Autodesk Inventor part; units mm, degrees
ref_plane "YZ Plane" through (0, 0, 0) normal (1, 0, 0) x (0, 1, 0)
ref_plane "XZ Plane" through (0, 0, 0) normal (0, 1, 0) x (-1, 0, 0)
ref_plane "XY Plane" through (0, 0, 0) normal (0, 0, 1) x (1, 0, 0)
sketch "스케치1" plane through (0, 0, 0) normal (0, 1, 0) x (-1, 0, 0)
  line L0 (0, 0) -> (-315, 0)
  line L1 (-315, 0) -> (-315, -950)
  line L2 (-315, -950) -> (0, -950)
  line L3 (0, -950) -> (0, 0)
  line L4 (-315, -645) -> (-315, -475)
  line L5 (-315, -475) -> (-535, -475)
  line L6 (-535, -475) -> (-535, -645)
  line L7 (-535, -645) -> (-315, -645)
  line L8 (-315, -645) -> (-315, -475)
  line L9 (-315, -475) -> (-535, -475)
  line L10 (-315, -305) -> (-315, -475)
  line L11 (-315, -475) -> (-535, -475)
  line L12 (-535, -475) -> (-535, -305)
  line L13 (-535, -305) -> (-315, -305)
  line L14 (-315, -305) -> (-315, -475)
  line L15 (0, -305) -> (0, 0)
  line L16 (0, -645) -> (0, -950)
  line L17 (0, 0) -> (175, 0)
  line L18 (175, 0) -> (175, -950)
  line L19 (175, -950) -> (0, -950)
  line L20 (0, -950) -> (0, 0)
  line L21 (175, 0) -> (145, 0)
  line L22 (145, 0) -> (145, -950)
  line L23 (145, -950) -> (175, -950)
  line L24 (175, -950) -> (175, 0)
  line L25 (175, -475) -> (145, -475)
  line L26 (145, -475) -> (145, -645)
  line L27 (145, -645) -> (175, -645)
  line L28 (175, -645) -> (175, -475)
  line L29 (175, -475) -> (145, -475)
  line L30 (145, -475) -> (145, -305)
  line L31 (145, -305) -> (175, -305)
  line L32 (175, -305) -> (175, -475)
  line L33 (145, -645) -> (-315, -645)
  line L34 (-315, -645) -> (-315, -685)
  line L35 (-315, -685) -> (145, -685)
  line L36 (145, -685) -> (145, -645)
  line L37 (145, -305) -> (-315, -305)
  line L38 (-315, -305) -> (-315, -265)
  line L39 (-315, -265) -> (145, -265)
  line L40 (145, -265) -> (145, -305)
  line L41 (0, 0) -> (145, -265)
  line L42 (145, -685) -> (0, -950)
  dimension "d0" = 315
  dimension "d1" = 950
  dimension "d3" = 220
  dimension "d4" = 170
  dimension "d5" = 220
  dimension "d6" = 170
  dimension "d7" = 175
  dimension "d8" = 30
  dimension "d9" = 460
  dimension "d10" = 40
  dimension "d11" = 460
  dimension "d12" = 40
extrude "돌출1" add sketch "스케치1" along normal blind 20 contours L3 L39 L1 L0 | L41 L39 L3 | L39 L22 L37 L3 | L3 L37 L1 L39 | L37 L22 L33 L3 | L3 L33 L1 L37 | L31 L18 L25 L22 | L1 L5 L12 L13 | L33 L22 L35 L3 | L3 L35 L1 L33 | L25 L18 L27 L22 | L1 L7 L6 L5 | L35 L42 L3 | L3 L2 L1 L35
sketch "스케치2" plane through (535, 0, -305) normal (1, 0, 0) x (0, 0, -1)
  line L0 (0, 0) -> (340, 0)
  line L1 (340, 0) -> (340, 20)
  line L2 (0, 20) -> (340, 20)
  line L3 (0, 0) -> (0, 20)
  line L4 (0, 20) -> (340, 20)
  line L5 (340, 20) -> (340, 0)
  line L6 (340, 0) -> (0, 0)
  line L7 (0, 0) -> (0, 20)
  point P0 (-305, 0)
extrude "돌출2" add sketch "스케치2" along normal blind 315
sketch "스케치3" plane through (-175, 0, -645) normal (-1, 0, 0) x (0, 0, 1)
  line L0 (0, 0) -> (340, 0)
  line L1 (340, 0) -> (340, 20)
  line L2 (0, 20) -> (340, 20)
  line L3 (0, 0) -> (0, 20)
  line L4 (0, 20) -> (340, 20)
  line L5 (340, 20) -> (340, 0)
  line L6 (340, 0) -> (0, 0)
  line L7 (0, 0) -> (0, 20)
  point P0 (645, 0)
extrude "돌출3" add sketch "스케치3" along normal blind 505
properties part number "cover" material "고무"
CAD build for the part. Positions are in the model's coordinates, mm. Round coordinates to 2 decimals unless told otherwise and drop trailing zeros. Order: outer loops, then holes, each group sorted by start corner. A loop starts at its lowest first (then second) coordinate and runs counter-clockwise, first axis right, second up. Notation, with made-up numbers: (-17.5, -3.5) -> (-8.5, -3.5) arc R17 ccw to (-8.5, 15.5) -> close; hole circle Ø3 at (12.5, 76.25). An arc over 180 degrees is marked (long way). Write item = value, one per line. Start each with the question number.
(1) Cut at C-C, the plane z = -280.5. List the corners of the cut face in (x, y), then the cut area to 3 significant figures.
(2) Pin check, flat tips, straight feed: P1, Ø1, axis at x = -351, z = -638.5, coming from the -Y side; P2, Ø6, axis at x = -440, y = 5, coming from the +Z side; P3, Ø6, axis at x = -505.5, y = 9, coming from the -Z side; P4, Ø10, axis at y = 13, z = -819.5, coming from the +X side. Stop position of each tip, or through.
(3) Cut at B-B, the plane x = -448. List the corners of the cut face in (y, z).
(4) Cut at A-A, the plane y = 11.25. List the corners of the cut face in (x, z), then the cut area to 3 significant figures.
(5) Probe line 1 (Z direction, x = 663.5, y = 1); line 2 (X direction, y = 3, z = -130); line 3 (X direction, y = 19.25, z = -752). List the from-to ranges inside material, lowest first. Write a range as [from, to].
Model answer:
q1.outline = (-145, 0) -> (315, 0) -> (315, 20) -> (-145, 20) -> close
q1.area = 9,200 mm2
q2.P1 = 0
q2.P2 = -305
q2.P3 = -645
q2.P4 = 315
q3.outline = (0, -645) -> (20, -645) -> (20, -305) -> (0, -305) -> close
q4.outline = (-680, -645) -> (-145, -645) -> (-145, -685) -> (0, -950) -> (315, -950) -> (315, -645) -> (850, -645) -> (850, -305) -> (315, -305) -> (315, 0) -> (0, 0) -> (-145, -265) -> (-145, -305) -> (-680, -305) -> close
q4.area = 762,000 mm2
q5.line_1 = [-645, -305]
q5.line_2 = [-71.13, 315]
q5.line_3 = [-108.34, 315]
